Check sheet for the modelled part. Datum: model origin and axes. Units: mm. Round coordinates to 2 decimals unless told otherwise and drop trailing zeros. Loops run counter-clockwise (first coordinate to the right, second up) from the corner with the lowest first, then second, coordinate; pieces in that order, holes last. Notation, with made-up numbers: (-14, 72) - (30, 72) arc R14 ccw to (30, 90) - close; hole circle Ø8 at (52.5, 50.25). An arc over 180 degrees is marked (long way). Put each result on its own line as item: value. Start each with the question number.
Item 1: Section check C-C, the plane z = 0.25. Give the number of separate pieces and of enclosed holes in the cut face, and give its area (3 significant figures).
Item 2: Draft check along X on faces 1 (the cylindrical face through (9.013, -1.423, 0.376)), 2 (the cylindrical face through (9.27, -6.11, 0.38)), 3 (the cylindrical face through (-10.875, -2.241, 0.376)). Enter one of: pulls with the +X half, pulls with the -X half, needs draft (parallel to the pull), parting line crosses it, or undercut.
Item 3: Material ranges on line 1 along Y through (x, z) = (0, 0.3) (3 decimals); line 2 along X through (y, z) = (-1.5, 0.15); line 3 along X through (y, z) = (5.5, 0.3), recorded low to high.
Item 4: Section check A-A, the plane x = 0. Record the cut outline in (y, z) (3 decimals).
from build123d import *

# Parameters (mm, degrees)
SKETCH1_R           = 0.47625
SKETCH1_R_2         = 3.175
BOSS_EXTRUDE1_DEPTH = 0.762
BOSS_EXTRUDE2_START = -0.762
SKETCH2_R           = 11.103539479
BOSS_EXTRUDE2_DEPTH = 0.762


with BuildPart() as part:
    # Sketch1 → Boss-Extrude1 (new body)
    with BuildSketch(Plane.XY):
        with BuildLine():
            ThreePointArc((-2.039848362, 9.751221095), (-4.130378192, 9.88369568), (-6.129577027, 9.25834098))
            ThreePointArc((-6.129577027, 9.25834098), (-6.747337126, 8.674137968), (-6.975028685, 7.854944918))
            ThreePointArc((-6.975028685, 7.854944918), (-7.339372349, 6.47410056), (-8.33754517, 5.452763952))
            ThreePointArc((-8.33754517, 5.452763952), (-9.909445645, 4.068211113), (-10.880900197, 2.212373372))
            ThreePointArc((-10.880900197, 2.212373372), (-10.904630014, 1.362455548), (-10.4863749, 0.622194736))
            ThreePointArc((-10.4863749, 0.622194736), (-9.767600366, -0.61183955), (-9.751221095, -2.039848362))
            ThreePointArc((-9.751221095, -2.039848362), (-9.883695679, -4.130378205), (-9.258340968, -6.129577051))
            ThreePointArc((-9.258340968, -6.129577051), (-8.674137957, -6.747337133), (-7.854944918, -6.975028685))
            ThreePointArc((-7.854944918, -6.975028685), (-6.47410056, -7.339372349), (-5.452763952, -8.33754517))
            ThreePointArc((-5.452763952, -8.33754517), (-4.068210251, -9.909446321), (-2.212371278, -10.880900842))
            ThreePointArc((-2.212371278, -10.880900842), (-1.362454485, -10.90462975), (-0.622194736, -10.4863749))
            ThreePointArc((-0.622194736, -10.4863749), (0.61183955, -9.767600366), (2.039848362, -9.751221095))
            ThreePointArc((2.039848362, -9.751221095), (4.130377433, -9.883695772), (6.129575677, -9.258341694))
            ThreePointArc((6.129575677, -9.258341694), (6.747336732, -8.674138622), (6.975028685, -7.854944918))
            ThreePointArc((6.975028685, -7.854944918), (7.339372349, -6.47410056), (8.33754517, -5.452763952))
            ThreePointArc((8.33754517, -5.452763952), (9.909446191, -4.068210417), (10.880900717, -2.212371682))
            ThreePointArc((10.880900717, -2.212371682), (10.904629801, -1.36245469), (10.4863749, -0.622194736))
            ThreePointArc((10.4863749, -0.622194736), (9.767600366, 0.61183955), (9.751221095, 2.039848362))
            ThreePointArc((9.751221095, 2.039848362), (9.883695769, 4.130377457), (9.258341673, 6.129575719))
            ThreePointArc((9.258341673, 6.129575719), (8.674138602, 6.747336744), (7.854944918, 6.975028685))
            ThreePointArc((7.854944918, 6.975028685), (6.47410056, 7.339372349), (5.452763952, 8.33754517))
            ThreePointArc((5.452763952, 8.33754517), (4.068210359, 9.909446236), (2.212371542, 10.880900761))
            ThreePointArc((2.212371542, 10.880900761), (1.362454619, 10.904629783), (0.622194736, 10.4863749))
            ThreePointArc((0.622194736, 10.4863749), (-0.61183955, 9.767600366), (-2.039848362, 9.751221095))
        make_face()
        with Locations((-7.854944918, -5.387528685)):
            Circle(SKETCH1_R, mode=Mode.SUBTRACT)
        with Locations((-1.167787514, -6.267444918)):
            Circle(SKETCH1_R, mode=Mode.SUBTRACT)
        with Locations((-5.257503273, -3.606002332)):
            Circle(SKETCH1_R, mode=Mode.SUBTRACT)
        with Locations(Location((0, 0, 0), (0, 0, 180))):
            Circle(SKETCH1_R_2, mode=Mode.SUBTRACT)
        with Locations((3.606002332, -5.257503273)):
            Circle(SKETCH1_R, mode=Mode.SUBTRACT)
        with Locations((5.387528685, -7.854944918)):
            Circle(SKETCH1_R, mode=Mode.SUBTRACT)
        with Locations((9.363842884, -1.744726751)):
            Circle(SKETCH1_R, mode=Mode.SUBTRACT)
        with Locations((6.267444918, -1.167787514)):
            Circle(SKETCH1_R, mode=Mode.SUBTRACT)
        with Locations((-9.363842884, 1.744726751)):
            Circle(SKETCH1_R, mode=Mode.SUBTRACT)
        with Locations((-6.267444918, 1.167787514)):
            Circle(SKETCH1_R, mode=Mode.SUBTRACT)
        with Locations((-3.606002332, 5.257503273)):
            Circle(SKETCH1_R, mode=Mode.SUBTRACT)
        with Locations((-5.387528685, 7.854944918)):
            Circle(SKETCH1_R, mode=Mode.SUBTRACT)
        with Locations((5.257503273, 3.606002332)):
            Circle(SKETCH1_R, mode=Mode.SUBTRACT)
        with BuildLine():
            ThreePointArc((1.255023852, 6.735637063), (1.635979659, 6.180208581), (1.080551177, 5.799252774))
            ThreePointArc((1.080551177, 5.799252774), (0.69959537, 6.354681256), (1.255023852, 6.735637063))
        make_face(mode=Mode.SUBTRACT)
        with Locations((1.744726751, 9.363842884)):
            Circle(SKETCH1_R, mode=Mode.SUBTRACT)
        with Locations((7.854944918, 5.387528685)):
            Circle(SKETCH1_R, mode=Mode.SUBTRACT)
        with Locations((-1.744726751, -9.363842884)):
            Circle(SKETCH1_R, mode=Mode.SUBTRACT)
    extrude(amount=BOSS_EXTRUDE1_DEPTH)

    # Sketch2 → Boss-Extrude2 (add)
    with BuildSketch(Plane.XY.offset(0.762).offset(BOSS_EXTRUDE2_START)):
        Circle(SKETCH2_R)
        with BuildLine():
            ThreePointArc((8.267572946, 5.149721676), (9.364843608, 2.67807766), (9.740246185, 0))
            ThreePointArc((9.740246185, 0), (9.716357017, -0.681763934), (9.644806696, -1.360183646))
            ThreePointArc((9.644806696, -1.360183646), (9.788473946, -1.529082312), (9.840092885, -1.744726751))
            ThreePointArc((9.840092885, -1.744726751), (9.741789124, -2.034503739), (9.487460012, -2.204653776))
            ThreePointArc((9.487460012, -2.204653776), (8.163793491, -5.312708498), (5.858113138, -7.781703297))
            ThreePointArc((5.858113138, -7.781703297), (5.862360186, -7.818214708), (5.863778685, -7.854944918))
            ThreePointArc((5.863778685, -7.854944918), (5.625812627, -8.267297711), (5.149721676, -8.267572946))
            ThreePointArc((5.149721676, -8.267572946), (2.016021533, -9.529325943), (-1.360183646, -9.644806696))
            ThreePointArc((-1.360183646, -9.644806696), (-1.831963088, -9.832035029), (-2.204653776, -9.487460012))
            ThreePointArc((-2.204653776, -9.487460012), (-5.312708498, -8.163793491), (-7.781703297, -5.858113138))
            ThreePointArc((-7.781703297, -5.858113138), (-8.247692164, -5.656905119), (-8.267572946, -5.149721676))
            ThreePointArc((-8.267572946, -5.149721676), (-9.529325943, -2.016021533), (-9.644806696, 1.360183646))
            ThreePointArc((-9.644806696, 1.360183646), (-9.832035029, 1.831963088), (-9.487460012, 2.204653776))
            ThreePointArc((-9.487460012, 2.204653776), (-8.163793491, 5.312708498), (-5.858113138, 7.781703297))
            ThreePointArc((-5.858113138, 7.781703297), (-5.656905119, 8.247692164), (-5.149721676, 8.267572946))
            ThreePointArc((-5.149721676, 8.267572946), (-2.016021533, 9.529325943), (1.360183646, 9.644806696))
            ThreePointArc((1.360183646, 9.644806696), (1.831963088, 9.832035029), (2.204653776, 9.487460012))
            ThreePointArc((2.204653776, 9.487460012), (5.312708498, 8.163793491), (7.781703297, 5.858113138))
            ThreePointArc((7.781703297, 5.858113138), (8.164729311, 5.74925744), (8.331194918, 5.387528685))
            ThreePointArc((8.331194918, 5.387528685), (8.315014565, 5.264443421), (8.267572946, 5.149721676))
        make_face(mode=Mode.SUBTRACT)
    extrude(amount=BOSS_EXTRUDE2_DEPTH)


solid = part.part
Check result:
1. separate pieces: 1
1. enclosed holes: 17
1. area: 344 mm²
2. face 1: undercut
2. face 2: pulls with the +X half
2. face 3: pulls with the -X half
3. line 1: -11.104 to -3.175, 3.175 to 11.104
3. line 2: -11 to -2.8, 2.8 to 5.93, 6.61 to 8.96, 9.77 to 11
3. line 3: -9.65 to -4.02, -3.2 to 7.39, 8.32 to 9.65
4. outline: (-11.104, 0) - (-3.175, 0) - (-3.175, 0.762) - (-11.104, 0.762) - close; (3.175, 0) - (11.104, 0) - (11.104, 0.762) - (3.175, 0.762) - close
